Check sheet for the drawn part. Datum: minimum x, y, z corner. Units: mm. A direction names the side the tool comes from. Round coordinates to 2 decimals unless told otherwise and drop trailing zeros. Write each loop counter-clockwise with the first axis right and the second up, starting at its lowest first coordinate (ties: lowest second). Pieces come first, ordered by that corner, then holes.
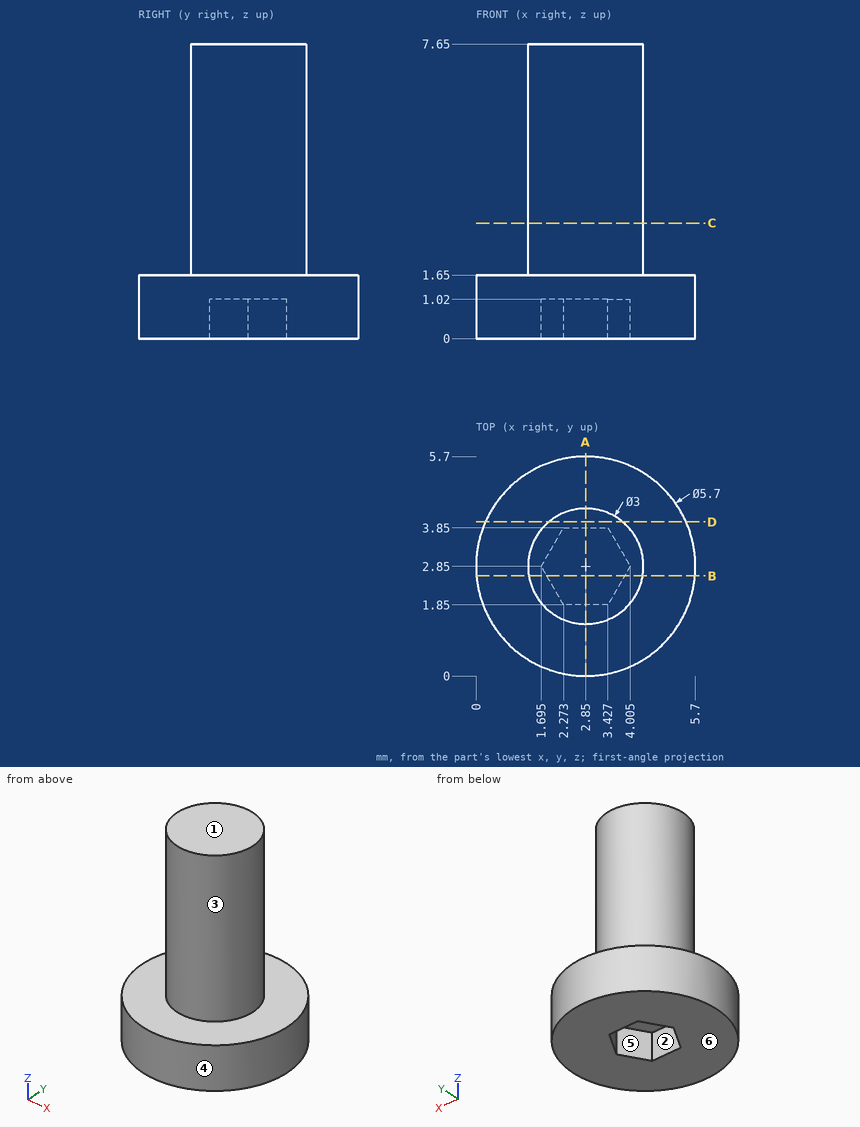
Q1. Sectioned sample at B-B (y = 2.6). Enter the section's corners in (x, z).
Recorded:
outline: (0.01, 0) - (1.84, 0) - (1.84, 1.02) - (3.86, 1.02) - (3.86, 0) - (5.69, 0) - (5.69, 1.65) - (4.33, 1.65) - (4.33, 7.65) - (1.37, 7.65) - (1.37, 1.65) - (0.01, 1.65) - close
Q2. Sectioned sample at C-C (z = 3). Enter the section's corners in (x, y).
Recorded:
outline: circle Ø3 at (2.85, 2.85)
Q3. Tool access check on the marked faces 1, 2 and 3. Record the directions out of +Z, -Z, +X, -X, +Y, -Y that give a thin tool (end or side, any length) a straight path to the whole face; none if there is none.
Recorded:
face 1: +Z, +X, -X, +Y, -Y
face 2: -Z
face 3: +Z
Q4. Sectioned sample at A-A (x = 2.85). Enter the section's corners in (y, z).
Recorded:
outline: (0, 0) - (1.85, 0) - (1.85, 1.02) - (3.85, 1.02) - (3.85, 0) - (5.7, 0) - (5.7, 1.65) - (4.35, 1.65) - (4.35, 7.65) - (1.35, 7.65) - (1.35, 1.65) - (0, 1.65) - close
Q5. Sectioned sample at D-D (y = 4). Enter the section's corners in (x, z).
Recorded:
outline: (0.24, 0) - (5.46, 0) - (5.46, 1.65) - (3.81, 1.65) - (3.81, 7.65) - (1.89, 7.65) - (1.89, 1.65) - (0.24, 1.65) - close
Q6. Release check for a two-part mould opening along X. For the marked faces 4, 5 and 6 record: released by +X, released by -X, zero draft, split by the parting line, or undercut.
Recorded:
face 4: split by the parting line
face 5: undercut
face 6: zero draft
Q7. Depth check by flat-ended pin: P1, Ø3, axis at x = 1.5, z = 4, coming from the +Y side; P2, Ø1.5, axis at x = 4.5, z = 4.5, coming from the +Y side; P3, Ø1.5, axis at x = 3.5, z = 4, coming from the -Y side. Enter the tip coordinate at first touch or a pass-through.
Recorded:
P1: stops at y = 4.35
P2: stops at y = 4.05
P3: stops at y = 1.35
Q8. Material ranges on line 1 along Z through (x, y) = (4.45, 5.1); line 2 along Y through (x, z) = (3.4, 6.25) (1 decimal); line 3 along X through (y, z) = (2.8, 3.5), recorded low to high.
Recorded:
line 1: z = 0 to 1.65
line 2: y = 1.5 to 4.2
line 3: x = 1.35 to 4.35
